The model under review builds one solid part; all positions refer to its coordinate system, in mm. Face numbers are marked on the shaded views. A direction names the side the tool comes from. Coordinates: 2 decimals unless noted, no trailing zeros. Write each loop counter-clockwise with the first axis right and the second up, starting at its lowest first coordinate (ties: lowest second). Pieces come first, ordered by that corner, then holes. Notation, with made-up numbers: (-36.75, 58) - (5.25, 58) arc R22 ccw to (5.25, 81) - close; hole circle Ø1 at (85.25, 29.5). An arc over 180 degrees is marked (long way). Put each result on its own line as item: value.
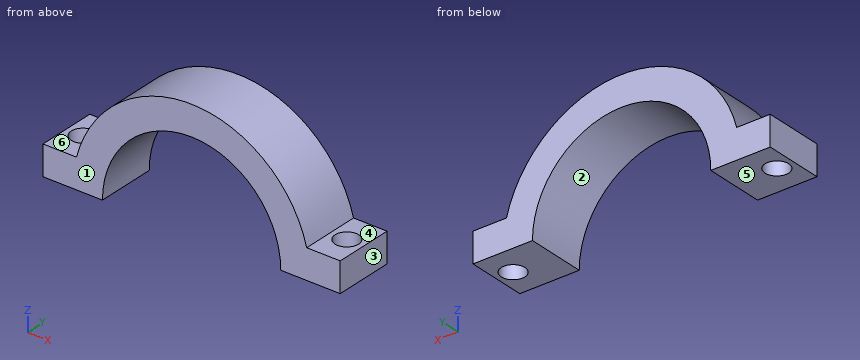
from build123d import *

# Parameters (mm, degrees)
F1_DEPTH = 12.7
F2_R     = 2.54
F3_DEPTH = 25.4
F4_R     = 2.54
F5_DEPTH = 25.4


with BuildPart() as f1:
    # F0 (on Front) → F1 (new body)
    with BuildSketch(Plane.XZ):
        with BuildLine():
            Line((-49.853401, 28.685216), (-49.853401, 22.335216))
            Line((-49.853401, 22.335216), (-43.503401, 22.335216))
            ThreePointArc((-43.503401, 22.335216), (-43.705847, 25.535725), (-44.309957, 28.685216))
            Line((-44.309957, 28.685216), (-49.853401, 28.685216))
        make_face()
        with BuildLine():
            ThreePointArc((-87.953401, 22.335216), (-68.903401, 41.385216), (-49.853401, 22.335216))
            Line((-49.853401, 22.335216), (-49.853401, 28.685216))
            Line((-49.853401, 28.685216), (-44.309957, 28.685216))
            ThreePointArc((-44.309957, 28.685216), (-68.903401, 47.735216), (-93.496846, 28.685216))
            Line((-93.496846, 28.685216), (-87.953401, 28.685216))
            Line((-87.953401, 28.685216), (-87.953401, 22.335216))
        make_face()
        with BuildLine():
            Line((-94.303401, 22.335216), (-87.953401, 22.335216))
            Line((-87.953401, 22.335216), (-87.953401, 28.685216))
            Line((-87.953401, 28.685216), (-93.496846, 28.685216))
            ThreePointArc((-93.496846, 28.685216), (-94.100956, 25.535725), (-94.303401, 22.335216))
        make_face()
        with BuildLine():
            ThreePointArc((-44.309957, 28.685216), (-43.705847, 25.535725), (-43.503401, 22.335216))
            Line((-43.503401, 22.335216), (-37.153401, 22.335216))
            Line((-37.153401, 22.335216), (-37.153401, 28.685216))
            Line((-37.153401, 28.685216), (-44.309957, 28.685216))
        make_face()
        with BuildLine():
            Line((-100.653401, 22.335216), (-94.303401, 22.335216))
            ThreePointArc((-94.303401, 22.335216), (-94.100956, 25.535725), (-93.496846, 28.685216))
            Line((-93.496846, 28.685216), (-100.653401, 28.685216))
            Line((-100.653401, 28.685216), (-100.653401, 22.335216))
        make_face()
    extrude(amount=F1_DEPTH)

    # F2 (on face) → F3 (cut)
    with BuildSketch(Plane.XY.offset(28.685216)):
        with Locations((-40.731679, -6.35)):
            Circle(F2_R)
    extrude(amount=-F3_DEPTH, mode=Mode.SUBTRACT)

    # F4 (on face) → F5 (cut)
    with BuildSketch(Plane.XY.offset(28.685216)):
        with Locations((-97.075124, -6.35)):
            Circle(F4_R)
    extrude(amount=-F5_DEPTH, mode=Mode.SUBTRACT)


solid = f1.part
1. Consider section C-C on y = -2.5. State the section outline as (x, z) points, plus the area to 3 significant figures.
Determined:
outline: (-100.65, 22.34) - (-87.95, 22.34) arc R19.05 cw to (-49.85, 22.34) - (-37.15, 22.34) - (-37.15, 28.69) - (-44.31, 28.69) arc R25.4 ccw to (-93.5, 28.69) - (-100.65, 28.69) - close
area: 527 mm^2
2. Consider section A-A on y = -6.35. State the section outline as (x, z) points, plus the area to 3 significant figures.
Determined:
outline: (-100.65, 22.34) - (-99.62, 22.34) - (-99.62, 28.69) - (-100.65, 28.69) - close; (-94.54, 22.34) - (-87.95, 22.34) arc R19.05 cw to (-49.85, 22.34) - (-43.27, 22.34) - (-43.27, 28.69) - (-44.31, 28.69) arc R25.4 ccw to (-93.5, 28.69) - (-94.54, 28.69) - close; (-38.19, 22.34) - (-37.15, 22.34) - (-37.15, 28.69) - (-38.19, 28.69) - close
area: 463 mm^2
3. Machinability: for the marked faces 4, 5 and 6, which of the approach directions +Z, -Z, +X, -X, +Y, -Y give a long, thin tool a straight path to every point of the face, cutting with its end or side? Answer none if there is none.
Determined:
face 4: +Z, +X, +Y, -Y
face 5: -Z, +X, -X, +Y, -Y
face 6: +Z, -X, +Y, -Y
4. To check wall thickness, follow probe 1 along X at (y, z) = (-8.75, 32); probe 2 along Z at (x, y) = (-44, -5.5); probe 3 along Y at (x, z) = (-96.5, 26). State the ranges of each line that lie inside material, in increasing order.
Determined:
probe 1: x = -92.39 to -85.32, -52.49 to -45.41
probe 2: z = 22.34 to 28.69
probe 3: y = -12.7 to -8.82, -3.88 to 0
5. For pin 1 Ø3 at (y, z) = (-6.5, 32) entering from -X; pin 2 Ø3 at (y, z) = (-4, 34) entering from +X; pin 3 Ø3 at (x, y) = (-61.5, -9.5) entering from +Z; pin 4 Ø10 at (x, z) = (-60.5, 37.5) entering from -Y, all flat-tipped, find the tip position at first contact; note any pin that passes through.
Determined:
pin 1: stops at x = -92.96
pin 2: stops at x = -45.63
pin 3: stops at z = 47.04
pin 4: stops at y = -12.7
6. The part is to be moulded in two halves that separate along X. For the marked faces 1, 2 and 3, say which applies: +X half, -X half, draft (parallel to the pull), parting line (faces both ways), or undercut.
Determined:
face 1: draft
face 2: undercut
face 3: +X half
7. Consider section D-D on z = 37.75. State the section outline as (x, y) points.
Determined:
outline: (-89.09, -12.7) - (-80.1, -12.7) - (-80.1, 0) - (-89.09, 0) - close; (-57.71, -12.7) - (-48.72, -12.7) - (-48.72, 0) - (-57.71, 0) - close
8. Consider section B-B on z = 33. State the section outline as (x, y) points, plus the area to 3 significant figures.
Determined:
outline: (-91.96, -12.7) - (-84.69, -12.7) - (-84.69, 0) - (-91.96, 0) - close; (-53.12, -12.7) - (-45.85, -12.7) - (-45.85, 0) - (-53.12, 0) - close
area: 185 mm^2
